Source: CAD feature listing. Evaluate the final solid. Frame: model axes, mm. Coordinates: 2 decimals unless noted, no trailing zeros. Order: outer loops, then holes, each group sorted by start corner. A loop starts at its lowest first (then second) coordinate and runs counter-clockwise, first axis right, second up. Notation, with made-up numbers: (-0.5, -34) -> (14.5, -34) arc R24 ccw to (14.5, -19) -> close; hole circle Ø10 at (82.5, 4). An arc over 180 degrees is marked (long way). Put each result on its own line as item: value.
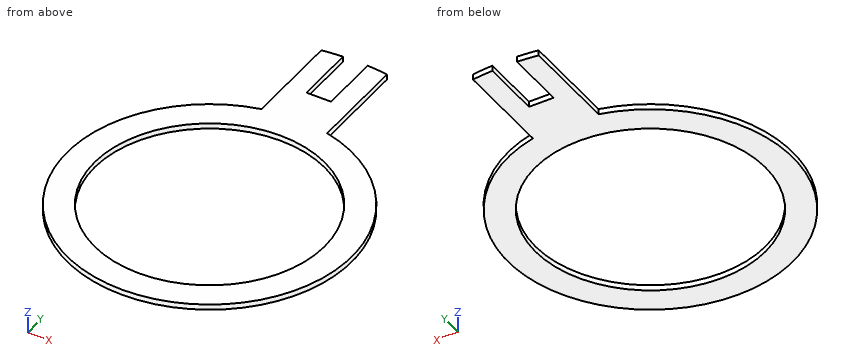
from build123d import *

# Parameters (mm, degrees)
SKETCH1_R           = 2.1
BOSS_EXTRUDE1_DEPTH = 0.1


with BuildPart() as part:
    # Sketch1 → Boss-Extrude1 (new body)
    with BuildSketch(Plane.XY):
        with BuildLine():
            Line((-0.6, 2.529822128), (-0.6, 4.318518264))
            ThreePointArc((-0.6, 4.318518264), (-0.412885429, 4.340406159), (-0.225, 4.35419051))
            Line((-0.225, 4.35419051), (-0.225, 3.26))
            Line((-0.225, 3.26), (0.225, 3.26))
            Line((0.225, 3.26), (0.225, 4.35419051))
            ThreePointArc((0.225, 4.35419051), (0.412885429, 4.340406159), (0.6, 4.318518264))
            Line((0.6, 4.318518264), (0.6, 2.529822128))
            ThreePointArc((0.6, 2.529822128), (0, -2.6), (-0.6, 2.529822128))
        make_face()
        Circle(SKETCH1_R, mode=Mode.SUBTRACT)
    extrude(amount=BOSS_EXTRUDE1_DEPTH)


solid = part.part
1. Cut plane C-C on y = 0. Output: boundary loops of the cut face in (x, z), plus the area to 4 significant figures.
Numbers:
outline: (-2.6, 0) -> (-2.1, 0) -> (-2.1, 0.1) -> (-2.6, 0.1) -> close; (2.1, 0) -> (2.6, 0) -> (2.6, 0.1) -> (2.1, 0.1) -> close
area: 0.1000 mm2
2. Ray query, line 1 along Y through (x, z) = (0.65, 0.05). Return the intervals inside material, ascending.
Numbers:
line 1: y = -2.52 to -2, 2 to 2.52
3. Cut plane B-B on z = 0.05. Output: boundary loops of the cut face in (x, y) (3 decimals).
Numbers:
outline: (-0.6, 2.53) arc R2.6 ccw (long way) to (0.6, 2.53) -> (0.6, 4.319) arc R4.36 ccw to (0.225, 4.354) -> (0.225, 3.26) -> (-0.225, 3.26) -> (-0.225, 4.354) arc R4.36 ccw to (-0.6, 4.319) -> close; hole circle Ø4.2 at (0, 0)
4. Cut plane D-D on y = 2.25. Output: boundary loops of the cut face in (x, z), plus the area to 3 significant figures.
Numbers:
outline: (-1.3, 0) -> (1.3, 0) -> (1.3, 0.1) -> (-1.3, 0.1) -> close
area: 0.261 mm2
5. Cut plane A-A on x = 0. Output: boundary loops of the cut face in (y, z).
Numbers:
outline: (-2.6, 0) -> (-2.1, 0) -> (-2.1, 0.1) -> (-2.6, 0.1) -> close; (2.1, 0) -> (3.26, 0) -> (3.26, 0.1) -> (2.1, 0.1) -> close
